Source: CAD feature listing. Evaluate the final solid. Frame: model axes, mm. Face numbers are marked on the shaded views. A direction names the side the tool comes from. Coordinates: 2 decimals unless noted, no trailing zeros. Order: outer loops, then holes, each group sorted by start corner. A loop starts at its lowest first (then second) coordinate and runs counter-clockwise, first axis right, second up. Notation, with made-up numbers: (52, 25.25) - (92, 25.25) arc R36 ccw to (92, 64.25) - close; hole circle Ø4 at (-17, 1.5). An arc over 180 degrees is marked (long way). One line per question, with ' | ' between items. Start each with the question number.
(1) Section D-D (y = -10.5). Return the cut outline in (x, z).
(2) Draft query along Y for the marked faces 1, 2 and 3. Return one class per face: +Y half, -Y half, draft (parallel to the pull), parting line (faces both ways), or undercut.
(3) Access query for the marked faces 4, 5 and 6. Directions: +Z, -Z, +X, -X, +Y, -Y. A direction counts if a zero-diameter tool reaches every point of the face in a straight line with its end or side. Return the directions, or none.
(4) Line query: line 1 along Y through (x, z) = (-39.5, 3); line 2 along Y through (x, z) = (-5, 12); line 3 along Y through (x, z) = (-8, 23). Output: solid intervals per line, ascending.
(5) Contact query for flat-ended pins moving along their axis: P1, Ø6, axis at x = -20, z = 20, coming from the -Y side; P2, Ø10, axis at y = 54, z = 21.5, coming from the +X side. Output: stop coordinate, or through.
(6) Section B-B (x = -5). Return the cut outline in (y, z).
(7) Section A-A (z = 20). Return the cut outline in (x, y).
(8) Section C-C (y = 32.5). Return the cut outline in (x, z), then the cut area to 3 significant figures.
from build123d import *

# Parameters (mm, degrees)
SKETCH1_R               = 4
BOSS_EXTRUDE1_DEPTH     = 40
CUT_EXTRUDE1_DEPTH      = 76.848533275
CUT_EXTRUDE1_DEPTH_BACK = 76.848533275
SKETCH3_R               = 2.5
CUT_EXTRUDE2_DEPTH      = 15


with BuildPart() as part:
    # Sketch1 → Boss-Extrude1 (new body)
    with BuildSketch(Plane.XY):
        Polygon((0, 0), (-40, 0), (-40, 20), (0, 20), (0, 45), (-40, 45), (-40, 65), (0, 65), (0, 68), (-43, 68), (-43, 65), (-43, 45), (-43, -18), (0, -18), align=None)
        with Locations((-35, 32.5)):
            Circle(SKETCH1_R, mode=Mode.SUBTRACT)
        with Locations((-5, 32.5)):
            Circle(SKETCH1_R, mode=Mode.SUBTRACT)
    extrude(amount=BOSS_EXTRUDE1_DEPTH)

    # Sketch3 → Cut-Extrude1 (cut, two sides: drawn at the far end of the back side and taken through both)
    with BuildSketch(Plane(origin=(0, 20, 0), x_dir=(-1, 0, 0), z_dir=(0, -1, 0)).offset(-CUT_EXTRUDE1_DEPTH_BACK)):
        with Locations(Location((20, -20, 0), (0, 0, 180))):
            Circle(SKETCH3_R)
    extrude(amount=CUT_EXTRUDE1_DEPTH + CUT_EXTRUDE1_DEPTH_BACK, mode=Mode.SUBTRACT)

    # Sketch4 → Cut-Extrude2 (cut)
    with BuildSketch(Plane(origin=(0, -18, 0), x_dir=(-1, 0, 0), z_dir=(0, -1, 0))):
        with BuildLine():
            Line((20, -24.25), (0, -24.25))
            Line((0, -24.25), (0, -15.75))
            Line((0, -15.75), (20, -15.75))
            ThreePointArc((20, -15.75), (24.25, -20), (20, -24.25))
        make_face()
    extrude(amount=-CUT_EXTRUDE2_DEPTH, mode=Mode.SUBTRACT)


solid = part.part
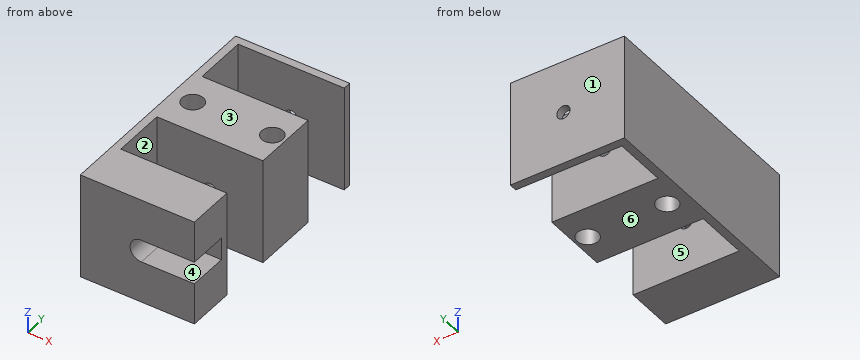
Response values:
1) outline: (-43, 0) - (0, 0) - (0, 15.75) - (-20, 15.75) arc R4.25 cw to (-20, 24.25) - (0, 24.25) - (0, 40) - (-43, 40) - close
2) face 1: +Y half | face 2: undercut | face 3: draft
3) face 4: +X, -Y | face 5: +Z, -Z, +X | face 6: -Z, +X, -X, +Y, -Y
4) line 1: y = -18 to 0, 20 to 45, 65 to 68 | line 2: y = -18 to 0, 20 to 28.5, 36.5 to 45, 65 to 68 | line 3: y = -3 to 0, 20 to 29.85, 35.15 to 45, 65 to 68
5) P1: stops at y = -3 | P2: stops at x = -40
6) outline: (-18, 0) - (0, 0) - (0, 40) - (-18, 40) - (-18, 24.25) - (-3, 24.25) - (-3, 15.75) - (-18, 15.75) - close; (20, 0) - (28.5, 0) - (28.5, 40) - (20, 40) - close; (36.5, 0) - (45, 0) - (45, 40) - (36.5, 40) - close; (65, 0) - (68, 0) - (68, 40) - (65, 40) - close
7) outline: (-43, -18) - (-24.25, -18) - (-24.25, -3) - (-22.5, -3) - (-22.5, 0) - (-40, 0) - (-40, 20) - (-22.5, 20) - (-22.5, 45) - (-40, 45) - (-40, 65) - (-22.5, 65) - (-22.5, 68) - (-43, 68) - close; (-17.5, -3) - (0, -3) - (0, 0) - (-17.5, 0) - close; (-17.5, 20) - (0, 20) - (0, 45) - (-17.5, 45) - close; (-17.5, 65) - (0, 65) - (0, 68) - (-17.5, 68) - close; hole circle Ø8 at (-35, 32.5); hole circle Ø8 at (-5, 32.5)
8) outline: (-43, 0) - (-39, 0) - (-39, 40) - (-43, 40) - close; (-31, 0) - (-9, 0) - (-9, 40) - (-31, 40) - close; (-1, 0) - (0, 0) - (0, 40) - (-1, 40) - close; hole circle Ø5 at (-20, 20) | area: 1,060 mm²
